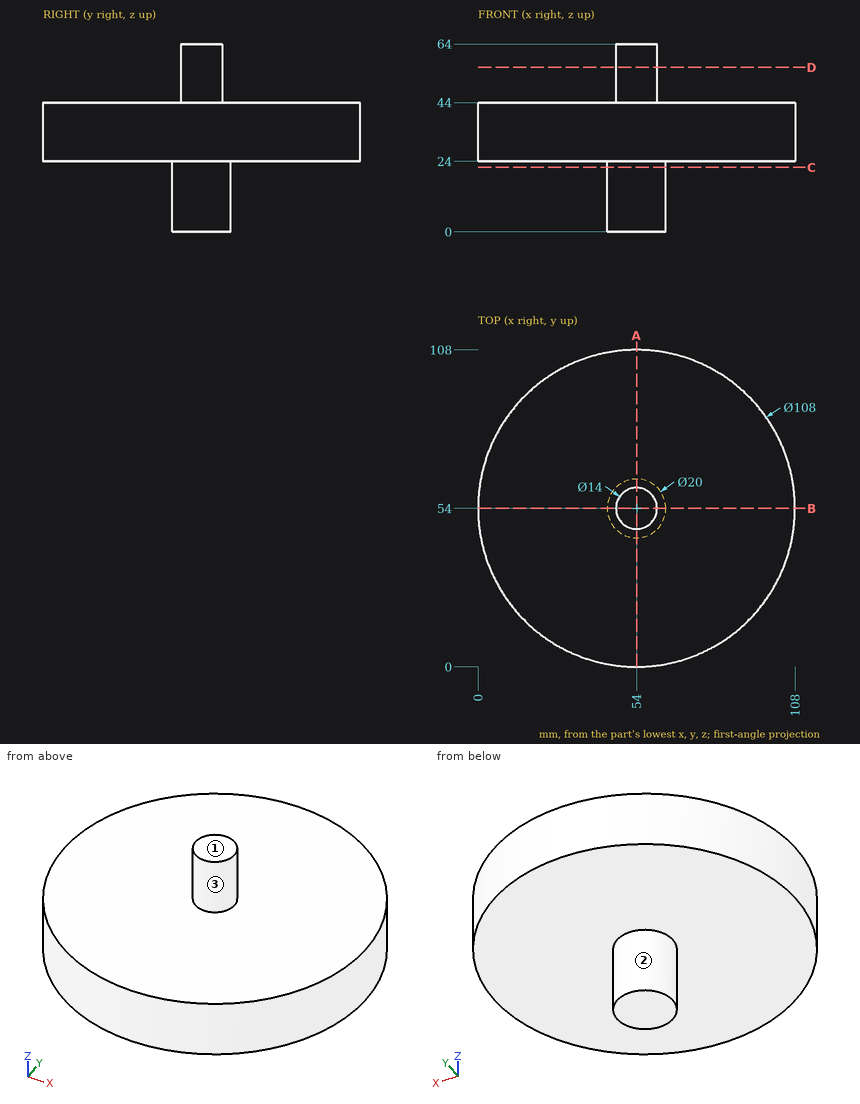
Geometry check sheet. Reference: drawing and pictorial views, mm from the part's lowest x, y, z. A direction names the side the tool comes from. Coordinates: 2 decimals unless noted, no trailing zeros. Loops run counter-clockwise (first coordinate to the right, second up) from the corner with the lowest first, then second, coordinate; pieces in that order, holes last.
1) Sectioned sample at A-A (x = 54). Record the boundary of the cut face in (y, z), and give its area (3 significant figures).
2) Material ranges on probe 1 along Z at (x, y) = (75.5, 83); probe 2 along Z at (x, y) = (47.5, 50); probe 3 along X at (y, z) = (55, 24.5), recorded low to high.
3) Access from +Z, -Z, +X, -X, +Y, -Y to the whole of each face (thin tool, end or side, straight path). Record for the marked faces 1, 2 and 3.
4) Sectioned sample at D-D (z = 56). Record the boundary of the cut face in (x, y).
5) Sectioned sample at C-C (z = 22). Record the boundary of the cut face in (x, y).
6) Gauge pin test, flat ends, axial feed: pin 1 (5 mm diameter, centred on x = 41, z = 20.5, fed in from +Y); pin 2 (2 mm diameter, centred on x = 56, z = 37.5, fed in from -Y); pin 3 (2 mm diameter, centred on y = 51.5, z = 55, fed in from +X); pin 4 (10 mm diameter, centred on x = 27, y = 21, fed in from +Z). Record the tip position at first contact, or that the pin passes through.
Check sheet entries:
1. outline: (0, 24) - (44, 24) - (44, 0) - (64, 0) - (64, 24) - (108, 24) - (108, 44) - (61, 44) - (61, 64) - (47, 64) - (47, 44) - (0, 44) - close
1. area: 2,920 mm2
2. probe 1: z = 24 to 44
2. probe 2: z = 0 to 44
2. probe 3: x = 0.01 to 107.99
3. face 1: +Z, +X, -X, +Y, -Y
3. face 2: -Z
3. face 3: +Z
4. outline: circle Ø14 at (54, 54)
5. outline: circle Ø20 at (54, 54)
6. pin 1: passes through
6. pin 2: stops at y = 0.01
6. pin 3: stops at x = 60.84
6. pin 4: stops at z = 44
